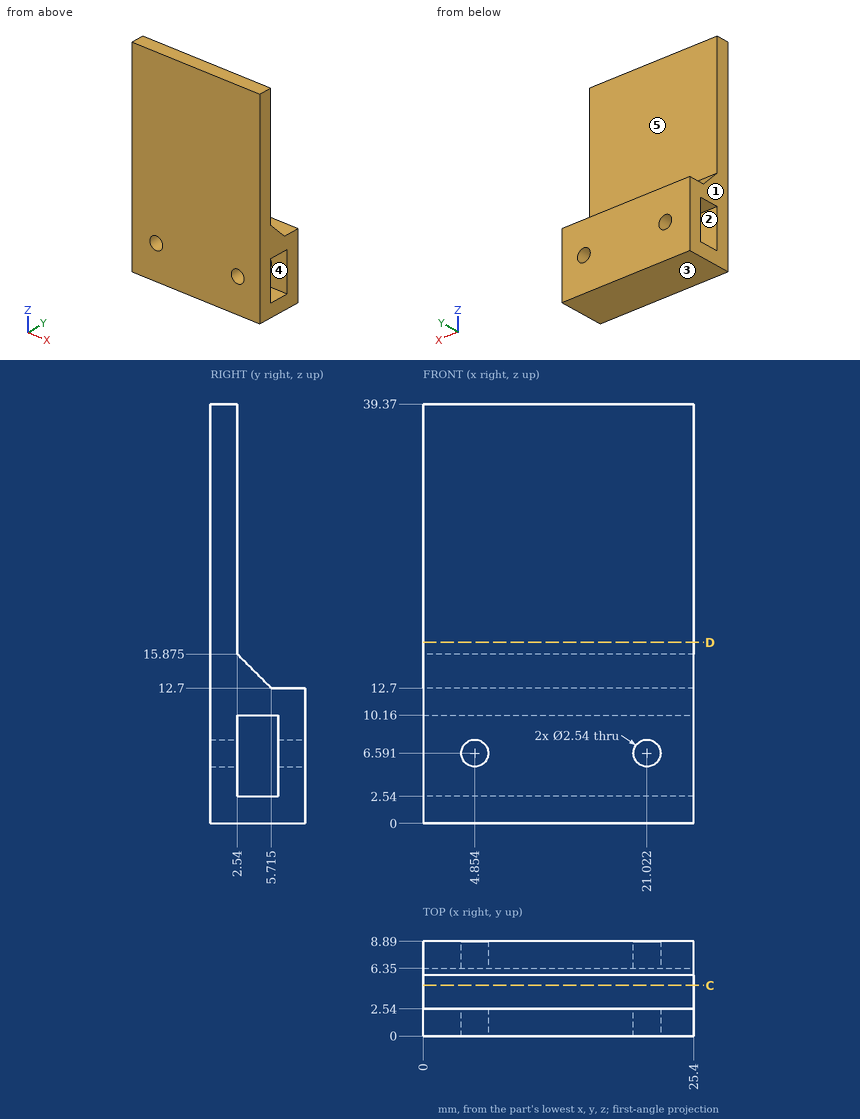
Design review of the part shown in the three views and the two pictorial views. Dimensions are in mm from the part's minimum x, y and z. A direction names the side the tool comes from. Round coordinates to 2 decimals unless told otherwise and drop trailing zeros. Order: outer loops, then holes, each group sorted by start corner. A loop starts at its lowest first (then second) coordinate and runs counter-clockwise, first axis right, second up. Notation, with made-up numbers: (33, 63.25) -> (65, 63.25) arc R20 cw to (65, 80.25) -> close; hole circle Ø8 at (-14, -12.5). An arc over 180 degrees is marked (long way). Write item = value, one per line. Start each with the question number.
1) To check wall thickness, follow line 1 (Z direction, x = 5, y = 1.25); line 2 (Y direction, x = 17.5, z = 26); line 3 (Z direction, x = 20.75, y = 3.25) (1 decimal). State the ranges of each line that lie inside material, in increasing order. Write a range as from..to.
2) Take a section at D-D on z = 17. State the section outline as (x, y) points.
3) Tool access review of the marked faces 1 and 2: name each direction out of +Z, -Z, +X, -X, +Y, -Y from which nothing blocks a thin tool from reaching the whole face with its end or side.
4) Insertion check: pin 1 (1.5 mm diameter, centred on x = 4.85, z = 6.59, fed in from -Y); pin 2 (3.5 mm diameter, centred on x = 12, y = 7, fed in from +Z) (1 decimal); pin 3 (2 mm diameter, centred on x = 16.5, z = 31, fed in from +Y). Each pin has a flat end and moves straight along its axis. Give the tip position at first contact, or say it passes through.
5) The part is to be moulded in two halves that separate along Y. For the marked faces 3, 4 and 5, say which applies: +Y half, -Y half, draft (parallel to the pull), parting line (faces both ways), or undercut.
6) Take a section at C-C on y = 4.75. State the section outline as (x, z) points (1 decimal).
Verdict:
q1.line_1 = 0..5.33, 7.85..39.37
q1.line_2 = 0..2.54
q1.line_3 = 0..2.5, 10.2..15.2
q2.outline = (0, 0) -> (25.4, 0) -> (25.4, 2.54) -> (0, 2.54) -> close
q3.face_1 = +Z, -Z, -X, +Y, -Y
q3.face_2 = +X, -X
q4.pin_1 = through
q4.pin_2 = 13.2
q4.pin_3 = 2.54
q5.face_3 = draft
q5.face_4 = undercut
q5.face_5 = +Y half
q6.outline = (0, 0) -> (25.4, 0) -> (25.4, 2.5) -> (0, 2.5) -> close; (0, 10.2) -> (25.4, 10.2) -> (25.4, 13.7) -> (0, 13.7) -> close
